```python
from build123d import *

# Parameters (mm, degrees)
CROQUIS1_W              = 82
CROQUIS1_H              = 5
SALIENTE_EXTRUIR1_DEPTH = 5
CROQUIS2_W              = 15
CROQUIS2_H              = 5
CROQUIS2_W_2            = 9
SALIENTE_EXTRUIR2_DEPTH = 22.4
CROQUIS3_W              = 8.993517989
CROQUIS3_H              = 5
CROQUIS3_W_2            = 10
SALIENTE_EXTRUIR3_DEPTH = 36
CROQUIS4_W              = 8.993517989
CROQUIS4_H              = 27.4
CROQUIS4_W_2            = 10
CROQUIS4_H_2            = 10
SALIENTE_EXTRUIR4_DEPTH = 5


with BuildPart() as part:
    # Croquis1 → Saliente-Extruir1 (new body)
    with BuildSketch(Plane.XY):
        with Locations((-17.772529993, -25.951946472)):
            Rectangle(CROQUIS1_W, CROQUIS1_H)
    extrude(amount=SALIENTE_EXTRUIR1_DEPTH)

    # Croquis2 → Saliente-Extruir2 (add)
    with BuildSketch(Plane(origin=(0, -23.451946472, 0), x_dir=(1, 0, 0), z_dir=(0, 1, 0))):
        with Locations((15.727470007, -2.5)):
            Rectangle(CROQUIS2_W, CROQUIS2_H)
        with Locations((-54.272529993, -2.5)):
            Rectangle(CROQUIS2_W_2, CROQUIS2_H)
    extrude(amount=SALIENTE_EXTRUIR2_DEPTH)

    # Croquis3 → Saliente-Extruir3 (add)
    with BuildSketch(Plane.XY.offset(5)):
        with Locations((-54.275770999, -25.951946472)):
            Rectangle(CROQUIS3_W, CROQUIS3_H)
        with Locations((-17.772529993, -25.951946472)):
            Rectangle(CROQUIS3_W_2, CROQUIS3_H)
        with Locations((18.227470007, -25.951946472)):
            Rectangle(CROQUIS3_W_2, CROQUIS3_H)
    extrude(amount=SALIENTE_EXTRUIR3_DEPTH)

    # Croquis4 → Saliente-Extruir4 (add)
    with BuildSketch(Plane.XY.offset(41)):
        with Locations((-54.275770999, -14.751946472)):
            Rectangle(CROQUIS4_W, CROQUIS4_H)
        with Locations((18.227470007, -23.451946472)):
            Rectangle(CROQUIS4_W_2, CROQUIS4_H_2)
    extrude(amount=SALIENTE_EXTRUIR4_DEPTH)


solid = part.part
```
Model file for the job. Use its own axes, mm. A direction names the side the tool comes from. Round coordinates to 2 decimals unless told otherwise and drop trailing zeros. Write each loop counter-clockwise with the first axis right and the second up, starting at its lowest first coordinate (ties: lowest second). Pieces come first, ordered by that corner, then holes. Notation, with made-up numbers: (84, 53.5) - (104, 53.5) arc R16 ccw to (104, 76.5) - close; hole circle Ø10 at (83.5, 13). An arc over 180 degrees is marked (long way). Use CSV: the item, a comma, the result in double quotes. Start each with the question number.
Item 1: Band-saw the part on A-A (z = 16). Write the cut outline in (x, y), and give its area (3 significant figures).
Item 2: Band-saw the part on D-D (x = -52.5). Write the cut outline in (y, z), and give its area (3 significant figures).
Item 3: Two-plate mould, pull along Z, no slides. Class faces 1 (the face through (-54, -23.452, 23)), 2 (the face through (18, -23, 46)), 3 (the face through (-12.773, -26, 23)): released by +Z, released by -Z, zero draft, split by the parting line, or undercut.
Item 4: Band-saw the part on B-B (y = -15). Write the cut outline in (x, z).
Item 5: Tool access for faces 4 (the face through (8.227, -12, 3)), 5 (the face through (-22.773, -26, 23)), 6 (the face through (18, -18.452, 43)): list every direction of +Z, -Z, +X, -X, +Y, -Y with a clear straight run to the whole face (end or side of a thin tool).
Item 6: Drill centre lines: L1, parallel to X at y = -26.5, z = 18.5; L2, parallel to Z at x = 19.5, y = -20.75; L3, parallel to X at y = -19.75, z = 43. Where is each one in solid material? Low to high. Write a range as [from, to].
Item 7: Band-saw the part on C-C (y = -19.25). Write the cut outline in (x, z).
Item 8: Pin check, flat tips, straight feed: P1, Ø10, axis at x = -32, y = -21.5, coming from the +Z side; P2, Ø7, axis at x = -56.5, z = 19, coming from the +Y side; P3, Ø5, axis at y = -19, z = 20, coming from the +X side; P4, Ø5, axis at y = -12, z = 40, coming from the +X side. Stop position of each tip, or through.
Checked values:
1,outline,"(-58.77, -28.45) - (-49.78, -28.45) - (-49.78, -23.45) - (-58.77, -23.45) - close; (-22.77, -28.45) - (-12.77, -28.45) - (-12.77, -23.45) - (-22.77, -23.45) - close; (13.23, -28.45) - (23.23, -28.45) - (23.23, -23.45) - (13.23, -23.45) - close"
1,area,"145 mm²"
2,outline,"(-28.45, 0) - (-1.05, 0) - (-1.05, 5) - (-23.45, 5) - (-23.45, 41) - (-1.05, 41) - (-1.05, 46) - (-28.45, 46) - close"
2,area,"454 mm²"
3,face 1,"undercut"
3,face 2,"released by +Z"
3,face 3,"zero draft"
4,outline,"(-58.77, 0) - (-49.77, 0) - (-49.77, 5) - (-58.77, 5) - close; (-58.77, 41) - (-49.78, 41) - (-49.78, 46) - (-58.77, 46) - close; (8.23, 0) - (23.23, 0) - (23.23, 5) - (8.23, 5) - close"
5,face 4,"+Z, -Z, +Y"
5,face 5,"+Z, +Y, -Y"
5,face 6,"+Z, +X, +Y"
6,L1,"x = [-58.77, -49.78], [-22.77, -12.77], [13.23, 23.23]"
6,L2,"z = [0, 5], [41, 46]"
6,L3,"x = [-58.77, -49.78], [13.23, 23.23]"
7,outline,"(-58.77, 0) - (-49.77, 0) - (-49.77, 5) - (-58.77, 5) - close; (-58.77, 41) - (-49.78, 41) - (-49.78, 46) - (-58.77, 46) - close; (8.23, 0) - (23.23, 0) - (23.23, 5) - (8.23, 5) - close; (13.23, 41) - (23.23, 41) - (23.23, 46) - (13.23, 46) - close"
8,P1,"stops at z = 5"
8,P2,"stops at y = -23.45"
8,P3,"passes through"
8,P4,"stops at x = -49.78"
